Design review of the part built by this model. Coordinates are the model's own, in mm. Give positions to 0.01 mm unless a question says otherwise; leave off trailing zeros. Loops run counter-clockwise (first coordinate to the right, second up) from the corner with the lowest first, then second, coordinate; pieces in that order, holes last. Notation, with made-up numbers: (26.25, 23) - (39.25, 23) arc R22 cw to (39.25, 54) - close; hole circle Ø5 at (-18.5, 37). An arc over 180 degrees is marked (long way). Write each question's results on one line, items separated by ' | '.
from build123d import *

# Parameters (mm, degrees)
SKETCH_1_W               = 147
SKETCH_1_H               = 37
EXTRUDE_1_DEPTH          = 2
SKETCH_2_R               = 1
CUT_EXTRUDE_604_DEPTH    = 2
SKETCH_5_R               = 1
SKETCH_5_R_2             = 32
FANS_DEPTH               = 10
CHAMFER_1_SIZE           = 4
SKETCH_6_W               = 44.721110511
SKETCH_6_H               = 34.816534288
SKETCH_6_W_2             = 53.357784661
SKETCH_6_W_3             = 25.346191928
SKETCH_6_H_2             = 23.882814665
CUT_EXTRUDE_1_DEPTH      = 10
HOLE_WIZARD_1_AT_2_COUNT = 2
HOLE_WIZARD_1_AT_2_PITCH = 61.5
HOLE_WIZARD_1_AT_3_COUNT = 2
HOLE_WIZARD_1_AT_3_PITCH = 71
HOLE_WIZARD_1_AT_4_COUNT = 2
HOLE_WIZARD_1_AT_4_PITCH = 132.5
HOLE_WIZARD_1_AT_5_COUNT = 2
HOLE_WIZARD_1_AT_5_PITCH = 140.023658715


with BuildPart() as part:
    # 草图1 → 凸台-拉伸1 (new body)
    with BuildSketch(Plane(origin=(0, 0, 0), x_dir=(1, 0, 0), z_dir=(0, 1, 0))):
        with Locations((73.5, -18.5)):
            Rectangle(SKETCH_1_W, SKETCH_1_H)
    extrude(amount=EXTRUDE_1_DEPTH)

    # 草图2 → Cut-Extrude 604 (cut)
    with BuildSketch(Plane(origin=(0, 2, 0), x_dir=(1, 0, 0), z_dir=(0, 1, 0))):
        with Locations(Location((144, -13, 0), (0, 0, 270))):
            Circle(SKETCH_2_R)
    extrude(amount=-CUT_EXTRUDE_604_DEPTH, mode=Mode.SUBTRACT)

    # 草图5 → Fans (cut)
    with BuildSketch(Plane(origin=(0, 2, 0), x_dir=(1, 0, 0), z_dir=(0, 1, 0))):
        with Locations(Location((75.25, -4.25, 0), (0, 0, 270))):
            Circle(SKETCH_5_R)
        with Locations(Location((136.75, -4.25, 0), (0, 0, 270))):
            Circle(SKETCH_5_R)
        with Locations((106, -35)):
            Circle(SKETCH_5_R_2)
        with Locations(Location((4.25, -4.25, 0), (0, 0, 270))):
            Circle(SKETCH_5_R)
        with Locations(Location((65.75, -4.25, 0), (0, 0, 270))):
            Circle(SKETCH_5_R)
        with Locations((35, -35)):
            Circle(SKETCH_5_R_2)
    extrude(amount=-FANS_DEPTH, mode=Mode.SUBTRACT)

    # 倒角1
    chamfer_1_edges = [part.edges().sort_by_distance(p)[0] for p in [
        (0, 1, 0),
        (147, 1, 0),
    ]]
    chamfer(chamfer_1_edges, length=CHAMFER_1_SIZE)

    # 草图6 → 切除-拉伸1 (cut)
    with BuildSketch(Plane(origin=(0, 0, 0), x_dir=(-1, 0, 0), z_dir=(0, -1, 0))):
        with Locations((-9.242414788, -25.408267144)):
            Rectangle(SKETCH_6_W, SKETCH_6_H)
        with Locations((-130.712137278, -33.408267144)):
            Rectangle(SKETCH_6_W_2, SKETCH_6_H)
        with Locations((-72.793206756, -27.941407333)):
            Rectangle(SKETCH_6_W_3, SKETCH_6_H_2)
    extrude(amount=-CUT_EXTRUDE_1_DEPTH, mode=Mode.SUBTRACT)

    # 草图8 → 打孔尺寸(%根据)内六角花形沉头螺钉的类型1 (revolve, cut)
    with BuildSketch(Plane(origin=(4.25, 2, 4.25), x_dir=(0, 0, 1), z_dir=(1, 0, 0))):
        Polygon((0, 0), (0, 2), (1.1, 2), (1.1, 1.1), (2.2, 0), align=None)
    hole_wizard_1 = revolve(axis=Axis((4.25, 8.35, 4.25), (0, -1, 0)), mode=Mode.SUBTRACT)

    # 打孔尺寸(%根据)内六角花形沉头螺钉的类型1 at 2: 打孔尺寸(%根据)内六角花形沉头螺钉的类型1 ×2
    with Locations(*[(i * HOLE_WIZARD_1_AT_2_PITCH, 0, 0) for i in range(1, HOLE_WIZARD_1_AT_2_COUNT)]):
        add(hole_wizard_1, mode=Mode.SUBTRACT)

    # 打孔尺寸(%根据)内六角花形沉头螺钉的类型1 at 3: 打孔尺寸(%根据)内六角花形沉头螺钉的类型1 ×2
    with Locations(*[(i * HOLE_WIZARD_1_AT_3_PITCH, 0, 0) for i in range(1, HOLE_WIZARD_1_AT_3_COUNT)]):
        add(hole_wizard_1, mode=Mode.SUBTRACT)

    # 打孔尺寸(%根据)内六角花形沉头螺钉的类型1 at 4: 打孔尺寸(%根据)内六角花形沉头螺钉的类型1 ×2
    with Locations(*[(i * HOLE_WIZARD_1_AT_4_PITCH, 0, 0) for i in range(1, HOLE_WIZARD_1_AT_4_COUNT)]):
        add(hole_wizard_1, mode=Mode.SUBTRACT)

    # 打孔尺寸(%根据)内六角花形沉头螺钉的类型1 at 5: 打孔尺寸(%根据)内六角花形沉头螺钉的类型1 ×2
    with Locations(*[Vector(0.9980456251626064, 0, 0.062489439858123795) * (i * HOLE_WIZARD_1_AT_5_PITCH) for i in range(1, HOLE_WIZARD_1_AT_5_COUNT)]):
        add(hole_wizard_1, mode=Mode.SUBTRACT)


solid = part.part
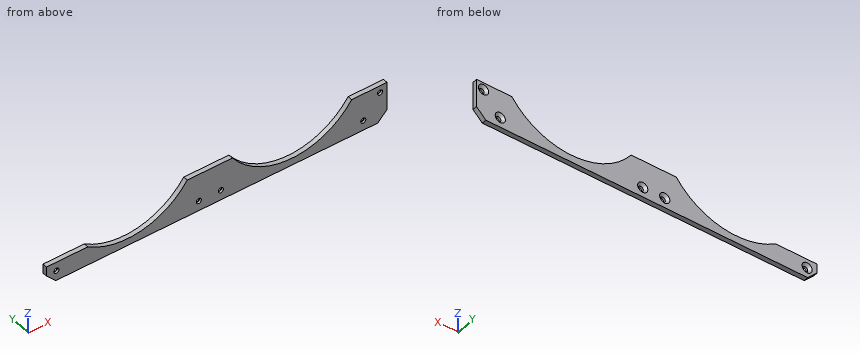
(1) Take a section at B-B on x = 51. Give the boundary of the cut face in (y, z), plus the area to 3 significant figures.
Answers below:
outline: (0, 0) - (2, 0) - (2, 7.29) - (0, 7.29) - close | area: 14.6 mm2
(2) Insertion check: P1, Ø1, axis at x = 106, y = 0.5, coming from the +Z side; P2, Ø3.5, axis at x = 4.25, z = 4.25, coming from the +Y side. Each pin has a flat end and moves straight along its axis. Give the tip position at first contact, or say it passes through.
Answers below:
P1: z = 3 | P2: y = 1.55
(3) Take a section at C-C on x = 103. Give the boundary of the cut face in (y, z).
Answers below:
outline: (0, 0) - (2, 0) - (2, 3.14) - (0, 3.14) - close
(4) Take a section at A-A on y = 0.3. Give the boundary of the cut face in (x, z), plus the area to 3 significant figures.
Answers below:
outline: (0, 4) - (4, 0) - (143, 0) - (147, 4) - (147, 16) - (131.75, 16) arc R32 cw to (80.25, 16) - (60.75, 16) arc R32 cw to (17.82, 8) - (0, 8) - close; hole circle Ø2.2 at (4.25, 4.25); hole circle Ø2.2 at (65.75, 4.25); hole circle Ø2.2 at (75.25, 4.25); hole circle Ø2.2 at (136.75, 4.25); hole circle Ø2.2 at (144, 13) | area: 1,280 mm2
(5) Wall thickness on line 1 along Z through (x, y) = (136.75, 0.55); line 2 along X through (y, z) = (0.5, 13); line 3 along Z through (x, y) = (4.25, 0.4): over which ranges is each line inside the solid? List them lowest first. Write a range as from..to.
Answers below:
line 1: 0..3.15, 5.35..16 | line 2: 58.24..82.76, 129.24..142.9, 145.1..147 | line 3: 0..3.15, 5.35..8
